Build history of the part. All positions in model axes, mm. Face numbers are marked on the shaded views. Round coordinates to 2 decimals unless told otherwise and drop trailing zeros. Write each loop counter-clockwise with the first axis right and the second up, starting at its lowest first coordinate (ties: lowest second). Pieces come first, ordered by that corner, then holes. Notation, with made-up numbers: M 63.25,44 L 101.25,44 A18 cw 101.25,50 Z; hole C -39,13 d10. An arc over 180 degrees is marked long. Write item = value, one per line. Start each with the question number.
Q1. Probe L1, parallel to Z at x = 0.4, y = 2.2; L2, parallel to Y at x = 2.1, z = 11; L3, parallel to X at y = -0.7, z = 12.5. List the from-to ranges inside material, lowest first.
Q2. Band-saw the part on C-C on z = 5.25. Write the cut outline in (x, y), plus the area to 3 significant figures.
Q3. Drop a flat-ended pin along its axis: P1, Ø1.5, axis at x = -2, z = 11, coming from the +Y side. Give the stop position or say it passes through.
Q4. Band-saw the part on D-D on z = 15.25. Write the cut outline in (x, y), plus the area to 3 significant figures.
Q5. Pull direction Z, two halves, no side cores. Call the marked faces 1, 2, 3 and 4: released by +Z, released by -Z, zero draft, split by the parting line, or undercut.
Q6. Band-saw the part on A-A on y = 0. Write the cut outline in (x, z).
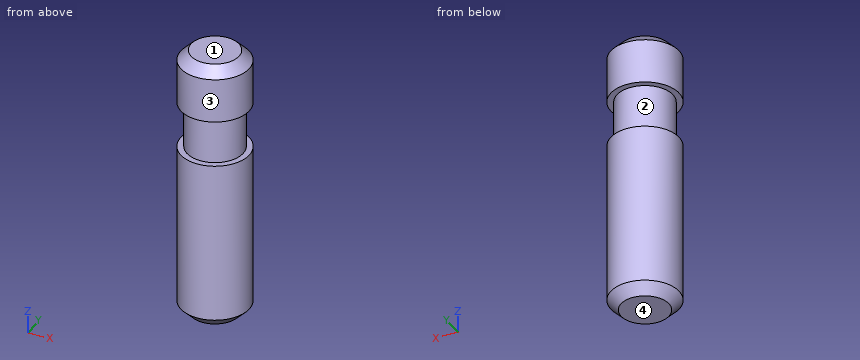
```python
from build123d import *

# Parameters (mm, degrees)
SKETCH_1_R      = 2.5
EXTRUDE_1_DEPTH = 20
CHAMFER_1_SIZE  = 0.75
SKETCH_2_W      = 3.4
SKETCH_2_H      = 0.45


with BuildPart() as part:
    # Sketch 1 → Extrude 1 (new body)
    with BuildSketch(Plane.XY):
        Circle(SKETCH_1_R)
    extrude(amount=EXTRUDE_1_DEPTH)

    # Chamfer 1
    chamfer_1_edges = [part.edges().sort_by_distance(p)[0] for p in [
        (-2.5, 0, 0),
        (-2.5, 0, 20),
    ]]
    chamfer(chamfer_1_edges, length=CHAMFER_1_SIZE)

    # Sketch 2 → Cut-Revolve 1 (revolve, cut)
    with BuildSketch(Plane(origin=(0, 0, 0), x_dir=(0, 0, -1), z_dir=(1, 0, 0)), mode=Mode.PRIVATE) as cut_revolve_1_sk:
        with Locations((-14.3, 2.275)):
            Rectangle(SKETCH_2_W, SKETCH_2_H)
    revolve(cut_revolve_1_sk.sketch.rotate(Axis((0, 0, 20), (0, 0, -1)), 90), axis=Axis((0, 0, 20), (0, 0, -1)), mode=Mode.SUBTRACT)


solid = part.part
```
Conclusion:
q1.L1 = 0.49 to 12.6, 16 to 19.51
q1.L2 = -1.36 to 1.36
q1.L3 = -2.4 to 2.4
q2.outline = C 0,0 d5
q2.area = 19.6 mm^2
q3.P1 = 2.17
q4.outline = C 0,0 d4.1
q4.area = 13.2 mm^2
q5.face_1 = released by +Z
q5.face_2 = undercut
q5.face_3 = zero draft
q5.face_4 = released by -Z
q6.outline = M -2.5,0.75 L -1.75,0 L 1.75,0 L 2.5,0.75 L 2.5,12.6 L 2.05,12.6 L 2.05,16 L 2.5,16 L 2.5,19.25 L 1.75,20 L -1.75,20 L -2.5,19.25 L -2.5,16 L -2.05,16 L -2.05,12.6 L -2.5,12.6 Z
